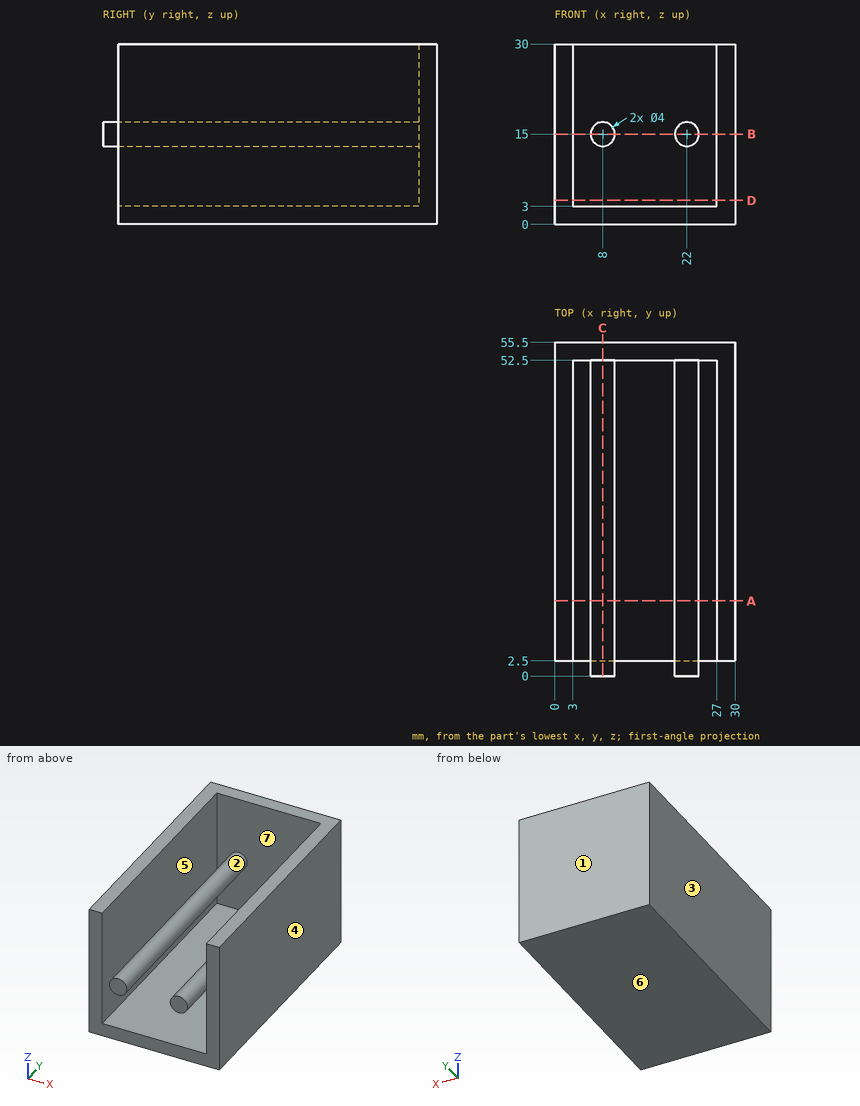
Part print with two shaded views. Sizes in mm from the minimum x, y, z corner. A direction names the side the tool comes from. Round coordinates to 2 decimals unless told otherwise and drop trailing zeros. Loops run counter-clockwise (first coordinate to the right, second up) from the corner with the lowest first, then second, coordinate; pieces in that order, holes last. Notation, with made-up numbers: M -24.5,55 L -15.5,55 A10 cw -15.5,66 Z; hole C 1.25,25.5 d2. An arc over 180 degrees is marked long. Return JSON: item names as keys, results as strings. Group by question number.
(1) Saw through at D-D, the plane z = 4. List the corners of the cut face in (x, y), and give its area (3 significant figures).
(2) Tool access for the marked faces 5, 6 and 7: list every direction of +Z, -Z, +X, -X, +Y, -Y with a clear straight run to the whole face (end or side of a thin tool).
(3) Mould opens along X. For the marked faces 1, 2, 3 and 4 say: +X half, -X half, draft (parallel to the pull), parting line (faces both ways), or undercut.
(4) Saw through at B-B, the plane z = 15. List the corners of the cut face in (x, y), and give its area (3 significant figures).
(5) Saw through at A-A, the plane y = 12.5. List the corners of the cut face in (x, z).
(6) Saw through at C-C, the plane x = 8. List the corners of the cut face in (y, z), and give its area (3 significant figures).
(7) Drop flat-ended pins along their axis: P1, Ø7, axis at x = 14.5, z = 12, coming from the -Y side; P2, Ø1.5, axis at x = 14.5, y = 17.5, coming from the +Z side; P3, Ø10, axis at x = 26.5, z = 24.5, coming from the -Y side. Give the stop position or say it passes through.
(8) Wall check: probe 1 along X at (y, z) = (48, 17.5); probe 2 along X at (y, z) = (23.5, 16.75); probe 3 along X at (y, z) = (49.5, 13.5). Give the ranges that are in metal, low to high. Write a range as [from, to].
Answer list:
{
 "1": {"outline": "M 0,2.5 L 3,2.5 L 3,52.5 L 27,52.5 L 27,2.5 L 30,2.5 L 30,55.5 L 0,55.5 Z", "area": "390 mm2"},
 "2": {"face 5": "+Z, -Y", "face 6": "-Z, +X, -X, +Y, -Y", "face 7": "-Y"},
 "3": {"face 1": "draft", "face 2": "undercut", "face 3": "-X half", "face 4": "+X half"},
 "4": {"outline": "M 0,2.5 L 3,2.5 L 3,52.5 L 6,52.5 L 6,0 L 10,0 L 10,52.5 L 20,52.5 L 20,0 L 24,0 L 24,52.5 L 27,52.5 L 27,2.5 L 30,2.5 L 30,55.5 L 0,55.5 Z", "area": "810 mm2"},
 "5": {"outline": "M 0,0 L 30,0 L 30,30 L 27,30 L 27,3 L 3,3 L 3,30 L 0,30 Z; C 8,15 d4; C 22,15 d4"},
 "6": {"outline": "M 0,13 L 52.5,13 L 52.5,3 L 2.5,3 L 2.5,0 L 55.5,0 L 55.5,30 L 52.5,30 L 52.5,17 L 0,17 Z", "area": "450 mm2"},
 "7": {"P1": "y = 52.5", "P2": "z = 3", "P3": "y = 2.5"},
 "8": {"probe 1": "[0, 3], [27, 30]", "probe 2": "[0, 3], [7.03, 8.97], [21.03, 22.97], [27, 30]", "probe 3": "[0, 3], [6.68, 9.32], [20.68, 23.32], [27, 30]"}
}
